```python
from build123d import *

# Parameters (mm, degrees)
SKETCH1_W           = 58
SKETCH1_H           = 24
SKETCH1_R           = 2.1
SKETCH1_W_2         = 40.4
SKETCH1_H_2         = 21.3
BOSS_EXTRUDE1_DEPTH = 28.35
SKETCH11_W          = 58
SKETCH11_H          = 24
BOSS_EXTRUDE5_DEPTH = 3.175
SKETCH14_W          = 24
SKETCH14_H          = 12
BOSS_EXTRUDE7_DEPTH = 10
CUT_EXTRUDE1_DEPTH  = 3.8
FILLET1_R           = 8
CHAMFER2_SIZE       = 3
CHAMFER3_SIZE       = 1
SKETCH19_W          = 8
SKETCH19_H          = 6
CUT_EXTRUDE3_DEPTH  = 2.75
SKETCH20_W          = 8.8
SKETCH20_H          = 8.5
CUT_EXTRUDE4_DEPTH  = 4
SKETCH21_W          = 20
SKETCH21_H          = 20
BOSS_EXTRUDE8_DEPTH = 6
SKETCH13_R          = 2.55
BOSS_EXTRUDE6_DEPTH = 5
FILLET4_R           = 1
CHAMFER4_SIZE       = 2
FILLET5_R           = 1
CUT_EXTRUDE5_REACH  = 77.835
SKETCH22_W          = 7
SKETCH22_H          = 7


with BuildPart() as part:
    # Sketch1 → Boss-Extrude1 (new body)
    with BuildSketch(Plane(origin=(0, 0, 0), x_dir=(1, 0, 0), z_dir=(0, 1, 0))):
        with Locations((29.95, -9.622651473)):
            Rectangle(SKETCH1_W, SKETCH1_H)
        with Locations(Location((55.15, -4.622651473, 0), (0, 0, 270))):
            Circle(SKETCH1_R, mode=Mode.SUBTRACT)
        with Locations(Location((55.15, -14.622651473, 0), (0, 0, 270))):
            Circle(SKETCH1_R, mode=Mode.SUBTRACT)
        with Locations(Location((4.75, -14.622651473, 0), (0, 0, 90))):
            Circle(SKETCH1_R, mode=Mode.SUBTRACT)
        with Locations(Location((4.75, -4.622651473, 0), (0, 0, 90))):
            Circle(SKETCH1_R, mode=Mode.SUBTRACT)
        with Locations((29.95, -9.622651473)):
            Rectangle(SKETCH1_W_2, SKETCH1_H_2, mode=Mode.SUBTRACT)
    extrude(amount=BOSS_EXTRUDE1_DEPTH)

    # Sketch11 → Boss-Extrude5 (add)
    with BuildSketch(Plane.XZ):
        with Locations((29.95, 9.622651473)):
            Rectangle(SKETCH11_W, SKETCH11_H)
    extrude(amount=BOSS_EXTRUDE5_DEPTH)

    # Sketch14 → Boss-Extrude7 (add)
    with BuildSketch(Plane(origin=(0, 0, -2.377348527), x_dir=(-1, 0, 0), z_dir=(0, 0, -1))):
        with Locations((-12.95, 12.5875)):
            Rectangle(SKETCH14_W, SKETCH14_H)
    extrude(amount=BOSS_EXTRUDE7_DEPTH)

    # Sketch16 → Cut-Extrude1 (cut, symmetric)
    with BuildSketch(Plane(origin=(0, 0, -7.377348527), x_dir=(-1, 0, 0), z_dir=(0, 0, -1))):
        with BuildLine():
            Line((-11.45, 16.7875), (-24.95, 16.7875))
            Line((-24.95, 16.7875), (-24.95, 8.3875))
            Line((-24.95, 8.3875), (-11.45, 8.3875))
            ThreePointArc((-11.45, 8.3875), (-7.25, 12.5875), (-11.45, 16.7875))
        make_face()
    extrude(amount=CUT_EXTRUDE1_DEPTH, both=True, mode=Mode.SUBTRACT)

    # Fillet1
    fillet1_edges = [part.edges().sort_by_distance(p)[0] for p in [
        (12.95, 6.5875, -2.377348527),
        (12.95, 18.5875, -2.377348527),
    ]]
    fillet(fillet1_edges, radius=FILLET1_R)

    # Chamfer2
    chamfer2_edges = [part.edges().sort_by_distance(p)[0] for p in [
        (0.95, 6.5875, -11.377348527),
        (0.95, 18.5875, -11.377348527),
        (58.95, 12.5875, 21.622651473),
        (0.95, 12.5875, 21.622651473),
        (0.95, 27.46875, -2.377348527),
        (0.95, -2.29375, -2.377348527),
        (0.95, 4.244354249, -4.720494277),
        (0.95, 20.930645751, -4.720494277),
    ]]
    chamfer(chamfer2_edges, length=CHAMFER2_SIZE)

    # Chamfer3
    chamfer3_edges = [part.edges().sort_by_distance(p)[0] for p in [
        (0.95, 12.5875, -12.377348527),
        (14.45, 18.5875, -12.377348527),
        (24.95, 12.5875, -12.377348527),
        (14.45, 6.5875, -12.377348527),
    ]]
    chamfer(chamfer3_edges, length=CHAMFER3_SIZE)

    # Sketch19 → Cut-Extrude3 (cut)
    with BuildSketch(Plane(origin=(0, 25.35, 0), x_dir=(1, 0, 0), z_dir=(0, 1, 0))):
        with Locations((4.95, -4.622651473)):
            Rectangle(SKETCH19_W, SKETCH19_H)
        with Locations((4.95, -14.622651473)):
            Rectangle(SKETCH19_W, SKETCH19_H)
        with Locations((54.95, -14.622651473)):
            Rectangle(SKETCH19_W, SKETCH19_H)
        with Locations((54.95, -4.622651473)):
            Rectangle(SKETCH19_W, SKETCH19_H)
    extrude(amount=-CUT_EXTRUDE3_DEPTH, mode=Mode.SUBTRACT)

    # Sketch20 → Cut-Extrude4 (cut)
    with BuildSketch(Plane(origin=(0, 0, 0), x_dir=(1, 0, 0), z_dir=(0, 1, 0))):
        with Locations((5.35, -9.622651473)):
            Rectangle(SKETCH20_W, SKETCH20_H)
    extrude(amount=CUT_EXTRUDE4_DEPTH, mode=Mode.SUBTRACT)

    # Sketch21 → Boss-Extrude8 (add)
    with BuildSketch(Plane.XZ.offset(3.175)):
        with Locations((20, 9.622651473)):
            Rectangle(SKETCH21_W, SKETCH21_H)
    extrude(amount=BOSS_EXTRUDE8_DEPTH)

    # Sketch13 → Boss-Extrude6 (add)
    with BuildSketch(Plane.XZ.offset(9.175)):
        with Locations(Location((20, 9.622651473, 0), (0, 0, 270))):
            Circle(SKETCH13_R)
    extrude(amount=BOSS_EXTRUDE6_DEPTH)

    # Fillet4
    fillet4_edges = [part.edges().sort_by_distance(p)[0] for p in [
        (10, -3.175, 9.622651473),
        (20, -3.175, -0.377348527),
        (30, -3.175, 9.622651473),
        (20, -3.175, 19.622651473),
    ]]
    fillet(fillet4_edges, radius=FILLET4_R)

    # Chamfer4
    chamfer4_edges = [part.edges().sort_by_distance(p)[0] for p in [
        (10, -9.175, 9.622651473),
        (20, -9.175, -0.377348527),
        (30, -9.175, 9.622651473),
        (20, -9.175, 19.622651473),
    ]]
    chamfer(chamfer4_edges, length=CHAMFER4_SIZE)

    # Fillet5
    fillet5_edges = [part.edges().sort_by_distance(p)[0] for p in [
        (20, -14.175, 12.172651473),
    ]]
    fillet(fillet5_edges, radius=FILLET5_R)

    # Cut-Extrude5: up to this face of the body (flat: up to its plane)
    cut_extrude5_end = Plane(part.part.faces().sort_by_distance((55.15, 0, 14.622651473))[0])
    # Sketch22 → Cut-Extrude5 (cut, up to the picked face)
    with BuildSketch(Plane(origin=(0, 28.35, 0), x_dir=(1, 0, 0), z_dir=(0, 1, 0)), mode=Mode.PRIVATE) as cut_extrude5_sk1:
        with Locations((6.25, -9.622651473)):
            Rectangle(SKETCH22_W, SKETCH22_H)
    cut_extrude5_tool1 = split(extrude(cut_extrude5_sk1.sketch, amount=-CUT_EXTRUDE5_REACH, mode=Mode.PRIVATE), bisect_by=cut_extrude5_end, keep=Keep.BOTH, mode=Mode.PRIVATE)
    add(cut_extrude5_tool1.solids().sort_by(Axis((6.25, 28.35, 9.622651), (0, -1, 0)))[0], mode=Mode.SUBTRACT)


solid = part.part
```
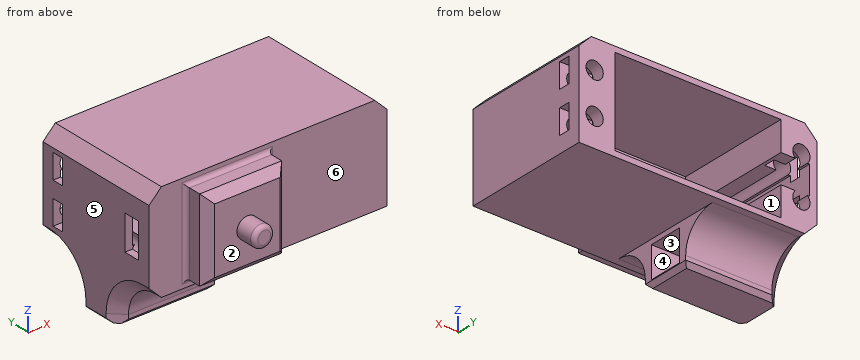
Work out the finished part from the listing and answer in its coordinate system (mm). Face numbers are marked on the shaded views. A direction names the side the tool comes from. Give positions to 0.01 mm unless a question says otherwise; leave off trailing zeros. Loops run counter-clockwise (first coordinate to the right, second up) from the corner with the lowest first, then second, coordinate; pieces in that order, holes last. Notation, with made-up numbers: (41.25, -23.75) - (50.25, -23.75) arc R16 ccw to (50.25, -18.75) - close; hole circle Ø3 at (10, 51.25). An arc over 180 degrees is marked (long way). Use CSV: the item, a comma, the result in double quotes. Start each with the question number.
(1) Find the intervals of material crossed by L1, parallel to Z at x = 55.15, y = 15.25; L2, parallel to X at y = 20.5, z = 1.5; L3, parallel to X at y = 18.5, z = 11, in increasing order.
(2) Determine the mould class of the marked faces 4, 5 and 6 for opening direction Y: released by +Y, released by -Y, zero draft, split by the parting line, or undercut.
(3) A tool of negligible diameter and unlimited length cuts with its end or side. For the marked faces 1, 2 and 3, from which of +Z, -Z, +X, -X, +Y, -Y can it reach the whole face along a straight path? Write none if from no direction.
(4) Find section C-C, the plane y = 13. Determine the outline of the cut face in (x, z).
(5) Each of these flat-tipped pins is pushed along its axis until it touches: pin 1 (5 mm diameter, centred on x = 51.5, y = 22, fed in from -Z); pin 2 (2.5 mm diameter, centred on x = 4.75, z = 14.62, fed in from +Y); pin 3 (1.5 mm diameter, centred on y = -7, z = 5, fed in from -X). Where does it stop, or does it pass through?
(6) Find section D-D, the plane z = 4.5. Count the separate pieces of the cut face and the enclosed holes in it, plus the area to 3 significant figures.
Results found:
1,L1,"-2.38 to 2.52, 6.72 to 12.52, 16.72 to 21.62"
1,L2,"0.95 to 9.75, 50.15 to 58.95"
1,L3,"0.95 to 2.75, 50.15 to 58.95"
2,face 4,"undercut"
2,face 5,"zero draft"
2,face 6,"released by -Y"
3,face 1,"+Y"
3,face 2,"-Y"
3,face 3,"+X"
4,outline,"(0.95, -11.38) - (1.95, -12.38) - (23.95, -12.38) - (24.95, -11.38) - (24.95, -11.18) - (7.27, -11.18) - (7.27, -3.58) - (24.95, -3.58) - (24.95, -2.38) - (58.95, -2.38) - (58.95, 18.62) - (55.95, 21.62) - (3.95, 21.62) - (0.95, 18.62) - close; hole (2.75, 6.12) - (3.28, 6.12) arc R2.1 ccw (long way) to (6.22, 6.12) - (9.75, 6.12) - (9.75, -1.03) - (50.15, -1.03) - (50.15, 20.27) - (9.75, 20.27) - (9.75, 13.12) - (6.22, 13.12) arc R2.1 ccw (long way) to (3.28, 13.12) - (2.75, 13.12) - close; hole circle Ø4.2 at (55.15, 4.62); hole circle Ø4.2 at (55.15, 14.62)"
5,pin 1,"z = -2.38"
5,pin 2,"y = 0"
5,pin 3,"x = 10"
6,separate pieces,"3"
6,enclosed holes,"0"
6,area,"541 mm^2"
